The figure shows three views and two pictorial views of one solid part (mm, origin at its lowest corner). Answer the questions. Give positions to 0.01 mm unless a question says otherwise; leave off trailing zeros. Loops run counter-clockwise (first coordinate to the right, second up) from the corner with the lowest first, then second, coordinate; pieces in that order, holes last. Notation, with made-up numbers: (-7.75, 44) - (17.25, 44) arc R22 ccw to (17.25, 58) - close; hole circle Ø8 at (5.5, 69.25). An arc over 180 degrees is marked (long way). Write item = value, one per line.
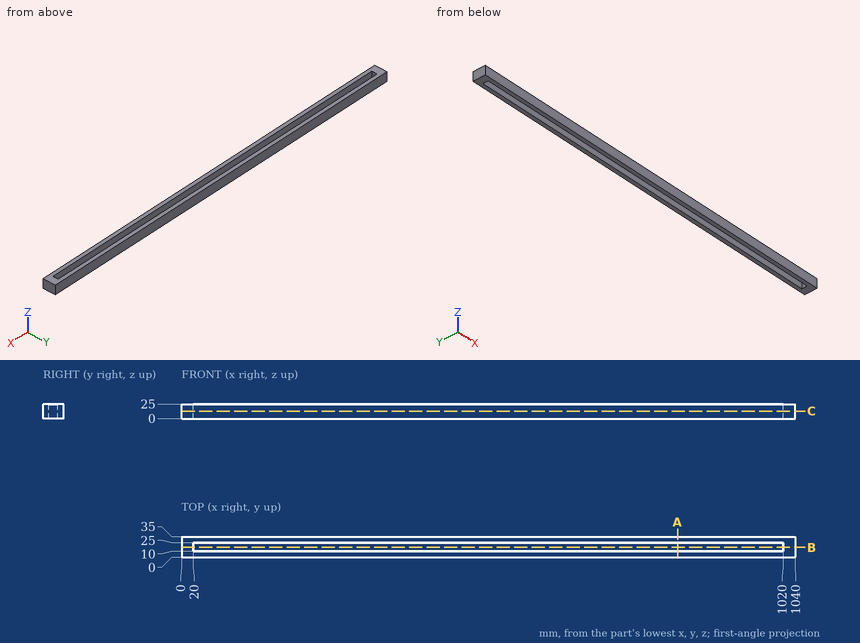
1) A cutting plane is placed at B-B on y = 17. Determine the outline of the cut face in (x, z).
Output:
outline = (0, 0) - (20, 0) - (20, 25) - (0, 25) - close; (1020, 0) - (1040, 0) - (1040, 25) - (1020, 25) - close
2) A cutting plane is placed at C-C on z = 12.75. Determine the outline of the cut face in (x, y), then the cut area to 3 significant figures.
Output:
outline = (0, 0) - (1040, 0) - (1040, 35) - (0, 35) - close; hole (20, 10) - (1020, 10) - (1020, 25) - (20, 25) - close
area = 21,400 mm²
3) Find the intervals of material crossed by probe 1 along X at (y, z) = (11.5, 18); probe 2 along Y at (x, z) = (67, 16), in increasing order.
Output:
probe_1 = 0 to 20, 1020 to 1040
probe_2 = 0 to 10, 25 to 35
4) A cutting plane is placed at A-A on x = 841. Determine the outline of the cut face in (y, z), then the cut area to 3 significant figures.
Output:
outline = (0, 0) - (10, 0) - (10, 25) - (0, 25) - close; (25, 0) - (35, 0) - (35, 25) - (25, 25) - close
area = 500 mm²
